Can you work these out from the model? Positions are in its coordinate system, mm. Coordinates: 2 decimals unless noted, no trailing zeros. Order: outer loops, then holes, each group sorted by start corner. A loop starts at its lowest first (then second) coordinate and runs counter-clockwise, first axis right, second up. Notation, with made-up numbers: (89, 69) - (128, 69) arc R27 ccw to (128, 107) - close; hole circle Ø5 at (26.5, -11.5). An arc over 180 degrees is marked (long way). Use a Markdown table: item, result. Add a question column.
(1) I want a section at A-A (y = 0). List the corners of the cut face in (x, z) for me (3 decimals), and give its area (3 significant figures).
(2) I want a section at C-C (x = -180). List the corners of the cut face in (y, z) for me (3 decimals).
(3) If I drill on L1, parallel to Y at x = -180, z = 1.7 (3 decimals); L2, parallel to Y at x = -214.5, z = 4.5; L3, parallel to X at y = -4, z = 0.45, over which ranges is the centre line in solid material (lowest first)? Write a range as [from, to].
(4) For pin 1 Ø2 at (x, z) = (113, 1.5) entering from -Y; pin 2 Ø1.5 at (x, z) = (174, 3.5) entering from +Y; pin 3 Ø2.5 at (y, z) = (-33.5, 3) entering from -X, each with a flat end and sliding along its axis, tell me the tip position at first contact or that it passes through.
(5) We'd pull the mould along X, two halves only. Please class faces 1 (the cylindrical face through (-184.92, 0.22, 2.54)), 2 (the flat face through (-4, 0, 0)): pulls with the +X half, pulls with the -X half, needs draft (parallel to the pull), parting line crosses it, or undercut.
(6) I want a section at B-B (z = 2.1). List the corners of the cut face in (x, y) for me (3 decimals).
Autodesk Inventor part; units mm, degrees
ref_plane "YZ Plane" through (0, 0, 0) normal (1, 0, 0) x (0, 1, 0)
ref_plane "XZ Plane" through (0, 0, 0) normal (0, 1, 0) x (-1, 0, 0)
ref_plane "XY Plane" through (0, 0, 0) normal (0, 0, 1) x (1, 0, 0)
sketch "Sketch1" plane through (0, 0, 0) normal (0, 0, 1) x (1, 0, 0)
  line L0 (-290, -30) -> (290, -30)
  line L1 (290, -30) -> (290, 30)
  line L2 (290, 30) -> (-290, 30)
  line L3 (-290, 30) -> (-290, -30)
  line L4 (-290, -30) -> (290, 30) construction
  line L5 (290, -30) -> (-290, 30) construction
  line L6 (-100, 35) -> (100, 35)
  line L7 (100, 35) -> (100, 30)
  line L8 (100, 30) -> (-100, 30)
  line L9 (-100, 30) -> (-100, 35)
  line L10 (-100, 35) -> (100, 30) construction
  line L11 (100, 35) -> (-100, 30) construction
  line L12 (-290, 0) -> (290, 0)
  line L13 (-100, -35) -> (100, -35)
  line L14 (100, -35) -> (100, -30)
  line L15 (100, -30) -> (-100, -30)
  line L16 (-100, -30) -> (-100, -35)
  line L17 (-100, -35) -> (100, -30) construction
  line L18 (100, -35) -> (-100, -30) construction
  point P0 (0, 0)
  point P1 (0, 32.5)
  point P2 (0, 30)
  point P3 (0, -32.5)
  point P4 (0, -30)
  point P5 (-100, 30)
  point P6 (-100, -30)
  dimension "d0" = 580
  dimension "d1" = 60
  dimension "d2" = 5
  dimension "d3" = 200
extrude "Plate1" add sketch "Sketch1" along normal blind 5
sketch "Sketch2" plane through (0, 0, 5) normal (0, 0, 1) x (1, 0, 0)
  circle A0 centre (-180, 0) radius 4.925
  point P0 (0, 0)
  dimension "d5" = 9.85
  dimension "d6" = 180
extrude "Cut1" cut sketch "Sketch2" against normal blind 5
equation "\"d7\" = Thickness"
equation "\"d4\" = Thickness"
equation "\"BendRadius\" = Thickness"
equation "\"BendReliefWidth\" = Thickness"
equation "\"BendReliefDepth\" = 0.5 * Thickness"
equation "\"TransitionRadius\" = BendRadius"
equation "\"JacobiRadiusSize\" = BendRadius"
equation "\"GapSize\" = Thickness"
properties part number "Table-Base Fixation ( Power Port )"
Answers follow:
| question | item | result |
|---|---|---|
| 1 | outline | (-290, 0) - (-184.925, 0) - (-184.925, 5) - (-290, 5) - close; (-175.075, 0) - (290, 0) - (290, 5) - (-175.075, 5) - close |
| 1 | area | 2,850 mm² |
| 2 | outline | (-30, 0) - (-4.925, 0) - (-4.925, 5) - (-30, 5) - close; (4.925, 0) - (30, 0) - (30, 5) - (4.925, 5) - close |
| 3 | L1 | y = [-30, -4.925], [4.925, 30] |
| 3 | L2 | y = [-30, 30] |
| 3 | L3 | x = [-290, -182.87], [-177.13, 290] |
| 4 | pin 1 | stops at y = -30 |
| 4 | pin 2 | stops at y = 30 |
| 4 | pin 3 | stops at x = -100 |
| 5 | face 1 | undercut |
| 5 | face 2 | needs draft |
| 6 | outline | (-290, -30) - (-100, -30) - (-100, -35) - (100, -35) - (100, -30) - (290, -30) - (290, 30) - (100, 30) - (100, 35) - (-100, 35) - (-100, 30) - (-290, 30) - close; hole circle Ø9.85 at (-180, 0) |
